from build123d import *

# Parameters (mm, degrees)
F0_W     = 50
F0_H     = 50
F0_W_2   = 40
F0_H_2   = 40
F1_DEPTH = 2250
F2_W     = 50
F2_H     = 50
F2_W_2   = 40
F2_H_2   = 40
F3_DEPTH = 580
F5_DEPTH = 2150


with BuildPart() as f1:
    # F0 (on Front) → F1 (new body)
    with BuildSketch(Plane.XZ):
        Rectangle(F0_W, F0_H)
        Rectangle(F0_W_2, F0_H_2, mode=Mode.SUBTRACT)
    extrude(amount=F1_DEPTH)

    # F2 (on face) → F3 (join)
    with BuildSketch(Plane(origin=(0, 0, -25), x_dir=(1, 0, 0), z_dir=(0, 0, -1))):
        with Locations((0, 25)):
            Rectangle(F2_W, F2_H)
        with Locations((0, 25)):
            Rectangle(F2_W_2, F2_H_2, mode=Mode.SUBTRACT)
        with Locations((0, 2225)):
            Rectangle(F2_W, F2_H)
        with Locations((0, 2225)):
            Rectangle(F2_W_2, F2_H_2, mode=Mode.SUBTRACT)
    extrude(amount=F3_DEPTH)

    # F4 (on face) → F5 (join, through all)
    with BuildSketch(Plane.XZ.offset(50)):
        Polygon((-20, -225), (-25, -225), (-25, -245), (25, -245), (25, -240), (-20, -240), align=None)
    extrude(amount=F5_DEPTH)


solid = f1.part
Design review of the part built by this model. Coordinates are the model's own, in mm. A direction names the side the tool comes from. Give positions to 0.01 mm unless a question says otherwise; leave off trailing zeros. Write each loop counter-clockwise with the first axis right and the second up, starting at its lowest first coordinate (ties: lowest second). Pieces come first, ordered by that corner, then holes. Notation, with made-up numbers: M 6,14.25 L 22,14.25 A13 ccw 22,30.25 Z; hole C -25.75,28.25 d2. An arc over 180 degrees is marked long. Return JSON: item names as keys, results as strings. Group by question number.
Item 1: Take a section at C-C (y = -1689). Give the boundary of the cut face in (x, z), plus the area to 4 significant figures.
Item 2: The part is to be moulded in two halves that separate along X. For faces 1 (the flat face through (0, -5, -311)), 2 (the flat face through (0, -2200, -422)), 3 (the flat face through (-25, -1120, -242)), 4 (the flat face through (0, -2205, -311)), say which applies: pulls with the +X half, pulls with the -X half, needs draft (parallel to the pull), parting line crosses it, or undercut.
Item 3: Wall thickness on line 1 along Y through (x, z) = (-15.5, -322); line 2 along Z through (x, y) = (-15, -446.5); line 3 along X through (y, z) = (-1085.5, -234): over which ranges is each line inside the solid? List them lowest first.
Item 4: Take a section at B-B (z = -466). Give the boundary of the cut face in (x, y).
Item 5: Tool access review of faces 5 (the flat face through (-20, -1109, 0)), 6 (the flat face through (0, -1110, -245)), 7 (the flat face through (20, -25, -311)), 8 (the flat face through (0, 0, -286)): name each direction out of +Z, -Z, +X, -X, +Y, -Y from which nothing blocks a thin tool from reaching the whole face with its end or side.
Item 6: Clearance check with flat-ended pins moving along their axes: pin 1 Ø5 at (x, y) = (8, -1522) entering from -Z; pin 2 Ø7.5 at (y, z) = (-1065.5, -234.5) entering from +X. State where each tip first meets the part, or that it passes through.
Item 7: Take a section at A-A (x = 2). Give the boundary of the cut face in (y, z).
Return value:
{
 "1": {"outline": "M -25,-245 L 25,-245 L 25,-240 L -20,-240 L -20,-225 L -25,-225 Z; M -25,-25 L 25,-25 L 25,25 L -25,25 Z; hole M -20,-20 L 20,-20 L 20,20 L -20,20 Z", "area": "1,225 mm2"},
 "2": {"face 1": "undercut", "face 2": "needs draft", "face 3": "pulls with the -X half", "face 4": "undercut"},
 "3": {"line 1": "y = -2250 to -2245, -2205 to -2200, -50 to -45, -5 to 0", "line 2": "z = -245 to -240, -25 to -20, 20 to 25", "line 3": "x = -25 to -20"},
 "4": {"outline": "M -25,-2250 L 25,-2250 L 25,-2200 L -25,-2200 Z; M -25,-50 L 25,-50 L 25,0 L -25,0 Z; hole M -20,-2245 L 20,-2245 L 20,-2205 L -20,-2205 Z; hole M -20,-45 L 20,-45 L 20,-5 L -20,-5 Z"},
 "5": {"face 5": "+Y, -Y", "face 6": "-Z, +X, -X", "face 7": "-Z", "face 8": "+Z, -Z, +X, -X, +Y"},
 "6": {"pin 1": "stops at z = -245", "pin 2": "stops at x = -20"},
 "7": {"outline": "M -2250,-605 L -2245,-605 L -2245,-25 L -2205,-25 L -2205,-605 L -2200,-605 L -2200,-245 L -50,-245 L -50,-605 L -45,-605 L -45,-25 L -5,-25 L -5,-605 L 0,-605 L 0,-20 L -2250,-20 Z; M -2250,20 L 0,20 L 0,25 L -2250,25 Z; hole M -2200,-240 L -50,-240 L -50,-25 L -2200,-25 Z"}
}
